```python
from build123d import *

# Parameters (mm, degrees)
SZKIC1_W                       = 40
SZKIC1_H                       = 157.55
DODANIE_WYCI_GNI_CIE1_DEPTH    = 30
SZKIC2_W                       = 40
SZKIC2_H                       = 30
DODANIE_WYCI_GNI_CIE2_DEPTH    = 32
SZKIC3_R                       = 3
WYTNIJ_WYCI_GNI_CIE1_DEPTH     = 30
SFAZOWANIE1_SIZE               = 16
SZKIC4_R                       = 5.5
WYTNIJ_WYCI_GNI_CIE7_DEPTH     = 15
SFAZOWANIE2_SIZE               = 10
OTW_R_GWINTOWANY_M8X1_01_D     = 7
OTW_R_GWINTOWANY_M8X1_01_DEPTH = 21
OTW_R_GWINTOWANY_M8X1_01_TIP   = 2.103012167


with BuildPart() as part:
    # Szkic1 → Dodanie-wyciągnięcie1 (new body)
    with BuildSketch(Plane(origin=(0, 0, 0), x_dir=(1, 0, 0), z_dir=(0, 1, 0))):
        Rectangle(SZKIC1_W, SZKIC1_H)
    extrude(amount=DODANIE_WYCI_GNI_CIE1_DEPTH)

    # Szkic2 → Dodanie-wyciągnięcie2 (add)
    with BuildSketch(Plane(origin=(0, 0, 0), x_dir=(-1, 0, 0), z_dir=(0, -1, 0))):
        with Locations((0, 63.775)):
            Rectangle(SZKIC2_W, SZKIC2_H)
    extrude(amount=DODANIE_WYCI_GNI_CIE2_DEPTH)

    # Szkic3 → Wytnij-wyciągnięcie1 (cut)
    with BuildSketch(Plane(origin=(0, 30, 0), x_dir=(1, 0, 0), z_dir=(0, 1, 0))):
        with Locations(Location((-13, -73.775, 0), (0, 0, 270))):
            Circle(SZKIC3_R)
        with Locations(Location((13, -73.775, 0), (0, 0, 270))):
            Circle(SZKIC3_R)
        with Locations(Location((13, -21.775, 0), (0, 0, 270))):
            Circle(SZKIC3_R)
        with Locations(Location((-13, -21.775, 0), (0, 0, 270))):
            Circle(SZKIC3_R)
    extrude(amount=-WYTNIJ_WYCI_GNI_CIE1_DEPTH, mode=Mode.SUBTRACT)

    # Sfazowanie1
    # the kernel refuses this chamfer: 16 mm, written as the material it takes off along each edge
    with BuildSketch(Plane(origin=(61.146927807, 0, 78.775), x_dir=(0, 0.9996219169112968, 0.027495876610586494), z_dir=(-1, 0, 0))) as sfazowanie1_piece_1:
        Polygon((SFAZOWANIE1_SIZE * 0.999621916911, SFAZOWANIE1_SIZE * 0.0274958766106), (-SFAZOWANIE1_SIZE * 0.0274958766106, SFAZOWANIE1_SIZE * 0.999621916911), (0, 0), align=None)
    extrude(amount=122.293855615, mode=Mode.SUBTRACT)

    # Szkic4 → Wytnij-wyciągnięcie7 (cut)
    with BuildSketch(Plane.XZ):
        with Locations((13, 73.775)):
            Circle(SZKIC4_R)
        with Locations((-13, 73.775)):
            Circle(SZKIC4_R)
    extrude(amount=-WYTNIJ_WYCI_GNI_CIE7_DEPTH, mode=Mode.SUBTRACT)

    # Sfazowanie2
    sfazowanie2_edges = [part.edges().sort_by_distance(p)[0] for p in [
        (0, -32, -48.775),
    ]]
    chamfer(sfazowanie2_edges, length=SFAZOWANIE2_SIZE)

    # Otwór gwintowany M8x1.01
    with Locations(Plane(origin=(0, 0, -78.775), x_dir=(-1, 0, 0), z_dir=(0, 0, -1))):
        with Locations((-13, -25), (-13, 23), (13, 23), (13, -25)):
            Hole(OTW_R_GWINTOWANY_M8X1_01_D / 2, depth=OTW_R_GWINTOWANY_M8X1_01_DEPTH)
            with Locations((0, 0, -(OTW_R_GWINTOWANY_M8X1_01_DEPTH + OTW_R_GWINTOWANY_M8X1_01_TIP / 2))):  # 118° drill point
                Cone(0, OTW_R_GWINTOWANY_M8X1_01_D / 2, OTW_R_GWINTOWANY_M8X1_01_TIP, mode=Mode.SUBTRACT)


solid = part.part
```
Here's how the part is built. I have some questions about the finished solid (model axes, mm). A direction names the side the tool comes from. Round coordinates to 2 decimals unless told otherwise and drop trailing zeros. Order: outer loops, then holes, each group sorted by start corner. A loop starts at its lowest first (then second) coordinate and runs counter-clockwise, first axis right, second up. Notation, with made-up numbers: (27.25, 85.5) -> (81.25, 85.5) arc R16 ccw to (81.25, 112.5) -> close; hole circle Ø8 at (-33, 37). An arc over 180 degrees is marked (long way). Use a Markdown table: item, result. Add a question column.
(1) For pin 1 Ø6 at (x, y) = (6.5, -16.5) entering from +Z (3 decimals); pin 2 Ø10 at (x, z) = (-13, 73.775) entering from -Y; pin 3 Ø9 at (x, y) = (-13, -25) entering from -Z (3 decimals); pin 4 Ø1.5 at (x, z) = (-1.5, -40) entering from -Y, each with a flat end and sliding along its axis, tell me the tip position at first contact or that it passes through.
(2) I need wall thicknesses on line 1 along Z through (x, y) = (-3, -13.5) (3 decimals); line 2 along Y through (x, z) = (-16, 40.5); line 3 along Z through (x, y) = (-3, 3.5) (3 decimals). Which ranges of each line are inside material? Lowest first, please.
(3) Suppose I cut it at C-C, the plane z = 2. Please give me the cut outline in (x, y).
(4) Suppose I cut it at B-B, the plane y = -18. Please give me the cut outline in (x, z) (3 decimals).
(5) For faces 1 (the face through (11.175, 22.605, 71.394)), 2 (the face through (12.816, 11.212, 68.278)), 3 (the face through (-13.46, 26.47, -68.13)), 4 (the face through (0, -11, -48.775)), which set-ups out of +Z, -Z, +X, -X, +Y, -Y let a thin tool reach every point of the face, with its end or its side?
(6) If we mould it in two halves opening along X, with no side actions, what happens to faces 5 (the face through (-14.825, 22.605, 71.394)), 6 (the face through (-20, 13, -16)), 7 (the face through (0, 30, -1))? For each: released by +X, released by -X, zero draft, split by the parting line, or undercut.
(7) Suppose I cut it at A-A, the plane y = 7.5. Please give me the cut outline in (x, z) (3 decimals), and give its area (3 significant figures).
Verdict:
| question | item | result |
|---|---|---|
| 1 | pin 1 | z = -48.775 |
| 1 | pin 2 | y = 15 |
| 1 | pin 3 | z = -78.775 |
| 1 | pin 4 | y = 0 |
| 2 | line 1 | -78.775 to -48.775 |
| 2 | line 2 | 0 to 30 |
| 2 | line 3 | -78.775 to 66.275 |
| 3 | outline | (-20, 0) -> (20, 0) -> (20, 30) -> (-20, 30) -> close |
| 4 | outline | (-20, -78.775) -> (20, -78.775) -> (20, -48.775) -> (-20, -48.775) -> close |
| 5 | face 1 | +Y, -Y |
| 5 | face 2 | -Y |
| 5 | face 3 | -Z |
| 5 | face 4 | +Z, +X, -X, -Y |
| 6 | face 5 | undercut |
| 6 | face 6 | released by -X |
| 6 | face 7 | zero draft |
| 7 | outline | (-20, -78.775) -> (20, -78.775) -> (20, 70.275) -> (17.243, 70.275) arc R5.5 cw to (8.757, 70.275) -> (-8.757, 70.275) arc R5.5 cw to (-17.243, 70.275) -> (-20, 70.275) -> close; hole circle Ø6 at (-13, 21.775); hole circle Ø6 at (13, 21.775) |
| 7 | area | 5,880 mm2 |
